Input: part model. Units: mm. Frame: model coordinates. Face numbers are marked on the shaded views. Coordinates: 2 decimals unless noted, no trailing zeros. Write each loop counter-clockwise with the first axis right and the second up, starting at its lowest first coordinate (ties: lowest second). Pieces come first, ordered by that corner, then holes. Notation, with made-up numbers: (30.5, 29) - (35.5, 29) arc R15 ccw to (35.5, 37) - close; hole circle Ø2 at (10, -5). An arc over 180 degrees is marked (long way). One line per question, with ' | ' between items. Start each with the question number.
1) Draft query along Z for the marked faces 1, 2, 3 and 4. Return one class per face: released by +Z, released by -Z, zero draft, split by the parting line, or undercut.
2) Section query D-D on z = -15. Return loops of the section in (x, y).
3) Line query: line 1 (Y direction, x = -25.6, z = 15.5); line 2 (Z direction, x = -19, y = -14); line 3 (Z direction, x = -25, y = 4). Output: solid intervals per line, ascending.
4) Section query C-C on z = 0. Return loops of the section in (x, y).
5) First-contact query: P1, Ø4.5, axis at y = -11, z = -15.5, coming from the +X side; P2, Ø1.5, axis at x = -16.5, z = 11.5, coming from the +Y side. Flat tips, straight axial feed; report the tip coordinate or a pass-through.
6) Section query B-B on y = 4.5. Return loops of the section in (x, z).
7) Section query A-A on x = 3.5. Return loops of the section in (y, z).
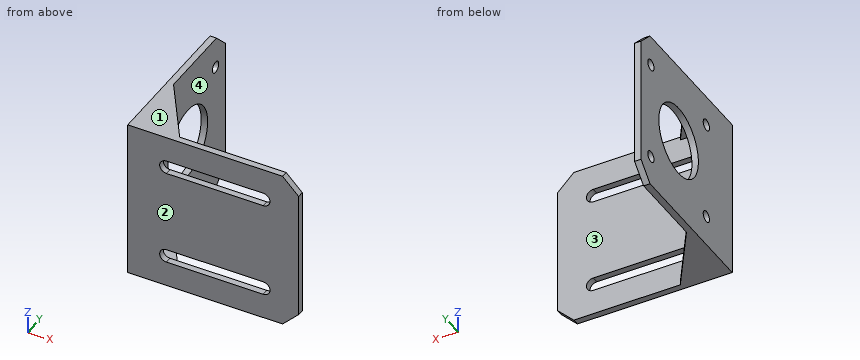
Autodesk Inventor part; units mm, degrees
ref_plane "YZ Plane" through (0, 0, 0) normal (1, 0, 0) x (0, 1, 0)
ref_plane "XZ Plane" through (0, 0, 0) normal (0, 1, 0) x (-1, 0, 0)
ref_plane "XY Plane" through (0, 0, 0) normal (0, 0, 1) x (1, 0, 0)
sketch "Sketch1" plane through (0, 0, 0) normal (0, 0, 1) x (1, 0, 0)
  line L0 (-26.5, 25.5) -> (-24.5, 25.5)
  line L1 (-24.5, 25.5) -> (-24.5, -23.5)
  line L2 (-26.5, -25.5) -> (26.5, -25.5)
  line L3 (26.5, -25.5) -> (26.5, -23.5)
  line L4 (26.5, -23.5) -> (-24.5, -23.5)
  line L5 (-26.5, 25.5) -> (-26.5, -25.5)
  point P0 (0, 0)
  point P1 (-26.5, 0)
  point P2 (0, -25.5)
  dimension "d1" = 51
  dimension "d2" = 2
  dimension "d4" = 2
  dimension "d5" = 53
extrude "Extrusion1" add sketch "Sketch1" along normal mid plane 50
sketch "Sketch2" plane through (-24.5, -23.5, 25) normal (1, 0, 0) x (0, 0, -1)
  circle A0 centre (25, 28) radius 11.05
  circle A1 centre (9.5, 43.5) radius 1.75
  circle A2 centre (40.5, 43.5) radius 1.75
  circle A3 centre (9.5, 12.5) radius 1.75
  circle A4 centre (40.5, 12.5) radius 1.75
  line L0 (0, 49) -> (50, 49)
  line L1 (9.5, 43.5) -> (40.5, 43.5) construction
  line L2 (9.5, 43.5) -> (9.5, 12.5) construction
  point P0 (25, 23.5)
  point P1 (25, 43.5)
  point P2 (9.5, 28)
  dimension "d8" = 22.1
  dimension "d9" = 3.5
  dimension "d10" = 31
  dimension "d11" = 31
  dimension "d12" = 21
extrude "Extrusion2" cut sketch "Sketch2" against normal up to next
sketch "Sketch3" plane through (-24.5, -23.5, 25) normal (1, 0, 0) x (0, 0, -1)
  line L0 (0, 44) -> (5, 49)
  line L1 (50, 49) -> (0, 49)
  line L2 (25, 22.7162) -> (25, 49) construction
  line L3 (50, 44) -> (45, 49)
  line L4 (0, 0) -> (0, 49)
  line L5 (50, 49) -> (50, 0)
  line L6 (0, 49) -> (50, 49)
  line L7 (45, 49) -> (50, 49)
  line L8 (50, 49) -> (50, 44)
  line L9 (5, 49) -> (0, 49)
  line L10 (0, 44) -> (0, 49)
  point P0 (25, 23.5)
  dimension "d15" = 45
  dimension "d16" = 5
extrude "Extrusion3" cut sketch "Sketch3" against normal up to next
sketch "Sketch4" plane through (-24.5, -23.5, 25) normal (0, 1, 0) x (1, 0, 0)
  arc A0 (10, 12.1) -> (10, 7.9) centre (10, 10) ccw
  arc A1 (10, 42.1) -> (10, 37.9) centre (10, 40) ccw
  arc A2 (40, 7.9) -> (40, 12.1) centre (40, 10) ccw
  arc A3 (40, 37.9) -> (40, 42.1) centre (40, 40) ccw
  line L0 (40, 7.9) -> (10, 7.9)
  line L1 (10, 12.1) -> (40, 12.1)
  line L2 (10, 37.9) -> (40, 37.9)
  line L3 (10, 42.1) -> (40, 42.1)
  line L4 (10, 10) -> (10, 40) construction
  line L5 (51, 50) -> (51, 0)
  point P0 (24.5, 25)
  point P1 (10, 25)
  dimension "d19" = 4.2
  dimension "d20" = 30
  dimension "d21" = 30
  dimension "d22" = 4.2
  dimension "d23" = 11
extrude "Extrusion4" cut sketch "Sketch4" against normal up to next
sketch "Sketch5" plane through (-24.5, -23.5, 25) normal (0, 1, 0) x (1, 0, 0)
  line L0 (10, 12.1) -> (40, 12.1)
  arc A0 (40, 7.9) -> (40, 12.1) centre (40, 10) ccw
  line L1 (40, 7.9) -> (10, 7.9)
  arc A1 (10, 12.1) -> (10, 7.9) centre (10, 10) ccw
  line L2 (40, 37.9) -> (10, 37.9)
  arc A2 (10, 42.1) -> (10, 37.9) centre (10, 40) ccw
  line L3 (10, 42.1) -> (40, 42.1)
  arc A3 (40, 37.9) -> (40, 42.1) centre (40, 40) ccw
  line L4 (0, 50) -> (0, 0)
  line L5 (51, 0) -> (0, 0)
  line L6 (51, 50) -> (51, 0)
  line L7 (0, 50) -> (51, 50)
  line L8 (46, 0) -> (51, 5)
  line L9 (51, 45) -> (46, 50)
  line L10 (51, 50) -> (-2, 50)
  point P0 (24.5, 25)
  dimension "d26" = 5
  dimension "d27" = 5
extrude "Extrusion5" cut sketch "Sketch5" against normal up to next contours L7 L6 L9 | L8 L6 L5
sketch "Sketch6" plane through (0, 0, 25) normal (0, 0, 1) x (1, 0, 0)
  line L0 (-11.5, -23.5) -> (-24.5, -3.5)
  line L1 (-11.5, -23.5) -> (-24.5, -23.5)
  line L2 (-24.5, -23.5) -> (-24.5, -3.5)
  point P0 (0, 0)
  dimension "d30" = 13
  dimension "d31" = 20
extrude "Extrusion6" add sketch "Sketch6" against normal blind 1
mirror "Mirror1" about plane through (0, 0, 0) normal (0, 0, 1) of "Extrusion6"
equation "\"d22\" = d19"
properties part number "mount-extruder"
Answer key:
1) face 1: released by +Z | face 2: zero draft | face 3: undercut | face 4: undercut
2) outline: (-26.5, -25.5) - (-16.6, -25.5) - (-16.6, -23.5) - (-24.5, -23.5) - (-24.5, -12.68) - (-26.5, -12.68) - close; (-26.5, -9.32) - (-24.5, -9.32) - (-24.5, 18.32) - (-26.5, 18.32) - close; (-26.5, 21.68) - (-24.5, 21.68) - (-24.5, 25.5) - (-26.5, 25.5) - close; (17.6, -25.5) - (26.5, -25.5) - (26.5, -23.5) - (17.6, -23.5) - close
3) line 1: -25.5 to -12.75, -9.25 to 18.25, 21.75 to 25.5 | line 2: -25 to -24, 24 to 25 | line 3: -25 to -11.04, 11.04 to 25
4) outline: (-26.5, -25.5) - (26.5, -25.5) - (26.5, -23.5) - (-24.5, -23.5) - (-24.5, -6.55) - (-26.5, -6.55) - close; (-26.5, 15.55) - (-24.5, 15.55) - (-24.5, 25.5) - (-26.5, 25.5) - close
5) P1: x = -24.5 | P2: y = -23.5
6) outline: (-26.5, -25) - (-24.5, -25) - (-24.5, -11.05) - (-26.5, -11.05) - close; (-26.5, 11.05) - (-24.5, 11.05) - (-24.5, 25) - (-26.5, 25) - close
7) outline: (-25.5, -25) - (-23.5, -25) - (-23.5, -17.1) - (-25.5, -17.1) - close; (-25.5, -12.9) - (-23.5, -12.9) - (-23.5, 12.9) - (-25.5, 12.9) - close; (-25.5, 17.1) - (-23.5, 17.1) - (-23.5, 25) - (-25.5, 25) - close
